Source: CAD feature listing. Evaluate the final solid. Frame: model axes, mm. A direction names the side the tool comes from. Coordinates: 2 decimals unless noted, no trailing zeros. Order: outer loops, then holes, each group sorted by start corner. A loop starts at its lowest first (then second) coordinate and runs counter-clockwise, first axis right, second up.
```python
from build123d import *

# Parameters (mm, degrees)
BOSS_EXTRUDE1_DEPTH      = 2.2
BOSS_EXTRUDE2_DEPTH      = 4.4
BOSS_EXTRUDE2_DEPTH_BACK = 2
SKETCH1_3_R              = 1.1
SKETCH2_R                = 0.7
BOSS_EXTRUDE3_DEPTH      = 0.6
BOSS_EXTRUDE3_TAPER      = 20


with BuildPart() as part:
    # Sketch1 → Boss-Extrude1 (new body)
    with BuildSketch(Plane(origin=(0, 0, 0), x_dir=(1, 0, 0), z_dir=(0, 1, 0))):
        with BuildLine():
            Line((3.782845085, 1.337043166), (3.527238547, 2.290979755))
            ThreePointArc((3.527238547, 2.290979755), (3.480645964, 2.35170039), (3.404764059, 2.361690433))
            Line((3.404764059, 2.361690433), (-0.362346663, 1.352296157))
            ThreePointArc((-0.362346663, 1.352296157), (-1.399770195, -0.025365361), (-0.313114699, -1.364536253))
            Line((-0.313114699, -1.364536253), (-0.385495815, -1.757932966))
            Line((-0.385495815, -1.757932966), (1.229595775, -1.466971493))
            Line((1.229595775, -1.466971493), (0.801769877, -2.8))
            Line((0.801769877, -2.8), (4.601769877, -2.8))
            ThreePointArc((4.601769877, -2.8), (4.884612589, -2.682842712), (5.001769877, -2.4))
            Line((5.001769877, -2.4), (5.001769877, -0.946410162))
            ThreePointArc((5.001769877, -0.946410162), (4.901769877, -0.773205081), (4.701769877, -0.773205081))
            Line((4.701769877, -0.773205081), (4.041625762, -1.154339463))
            ThreePointArc((4.041625762, -1.154339463), (3.81583188, -1.20709678), (3.598705744, -1.125718327))
            add(Edge.make_bspline(
                [(3.668101763, 0.674971994), (3.507811171, 0.443176193), (3.337919583, 0.271573974), (3.416349663, -0.986324141), (3.598705744, -1.125718327)],
                knots=[0.076223888, 0.076223888, 0.076223888, 0.076223888, 0.275181008, 0.474138129, 0.474138129, 0.474138129, 0.474138129], degree=3))
            ThreePointArc((3.668101763, 0.674971994), (3.798353982, 0.993376676), (3.782845085, 1.337043166))
        make_face()
    extrude(amount=BOSS_EXTRUDE1_DEPTH)

    # Sketch1<3> → Boss-Extrude2 (add, two sides: drawn at the far end of the back side and taken through both)
    with BuildSketch(Plane(origin=(0, 0, 0), x_dir=(1, 0, 0), z_dir=(0, 1, 0)).offset(-BOSS_EXTRUDE2_DEPTH_BACK)):
        with Locations(Location((0, 0, 0), (0, 0, 270))):
            Circle(SKETCH1_3_R)
    extrude(amount=BOSS_EXTRUDE2_DEPTH + BOSS_EXTRUDE2_DEPTH_BACK)

    # Sketch2 → Boss-Extrude3 (add)
    with BuildSketch(Plane.XY.offset(2.8)):
        with Locations((2.701769877, 1.2)):
            Circle(SKETCH2_R)
    extrude(amount=BOSS_EXTRUDE3_DEPTH, taper=BOSS_EXTRUDE3_TAPER)


solid = part.part
```
1. Draft query along Z for faces 5 (the flat face through (3.657, 1.085, -1.807)), 6 (the flat face through (1.02, 1.08, 2.12)), 7 (the flat face through (2, 2.2, 1)). Return one class per face: +Z half, -Z half, draft (parallel to the pull), parting line (faces both ways), or undercut.
2. Section query D-D, the plane z = 2.1. Output: boundary loops of the cut face in (x, y), plus the area to 3 significant figures.
3. Section query A-A, the plane x = -0.75. Output: boundary loops of the cut face in (y, z), plus the area to 3 significant figures.
4. Section query C-C, the plane y = 4. Output: boundary loops of the cut face in (x, z).
5. Section query B-B, the plane z = -1. Output: boundary loops of the cut face in (x, y).
6. Access query for faces 1 (the cylindrical face through (1.09, 3.28, -0.14)), 2 (the cylindrical face through (1.09, -1.01, -0.14)), 3 (the flat face through (0.411, 1.085, 1.614)), 4 (the flat face through (5.002, 1, 2)). Directions: +Z, -Z, +X, -X, +Y, -Y. A direction counts if a zero-diameter tool reaches every point of the face in a straight line with its end or side. Return the directions, or none.
7. Contact query for flat-ended pins moving along their axis: P1, Ø2.5, axis at x = 2.5, z = -1, coming from the -Y side; P2, Ø1.5, axis at x = 2.5, z = -0.5, coming from the +Y side; P3, Ø1.5, axis at x = 0, y = 0, coming from the +Z side. Output: stop coordinate, or through.
8. Material intervals for line 1 along Y through (x, z) = (2.5, 1.55); line 2 along Z through (x, y) = (0, -1.5); line 3 along X through (y, z) = (2, 1.1), sorted ascending.
Answer key:
1. face 5: -Z half
1. face 6: undercut
1. face 7: draft
2. outline: (1.03, 0) - (5, 0) - (5, 2.2) - (1.03, 2.2) - close
2. area: 8.75 mm2
3. outline: (-2, -0.8) - (0, -0.8) - (0, -1.18) - (2.2, -1.18) - (2.2, -0.8) - (4.4, -0.8) - (4.4, 0.8) - (2.2, 0.8) - (2.2, 1.18) - (0, 1.18) - (0, 0.8) - (-2, 0.8) - close
3. area: 12.0 mm2
4. outline: circle Ø2.2 at (0, 0)
5. outline: (-0.98, 0) - (-0.46, 0) - (-0.46, -2) - (0.46, -2) - (0.46, 0) - (3.8, 0) - (3.8, 2.2) - (0.46, 2.2) - (0.46, 4.4) - (-0.46, 4.4) - (-0.46, 2.2) - (-0.98, 2.2) - close
6. face 1: +Y
6. face 2: -Y
6. face 3: +Y, -Y
6. face 4: +Z, -Z, +X, +Y, -Y
7. P1: stops at y = 0
7. P2: stops at y = 2.2
7. P3: stops at z = 1.76
8. line 1: y = 0 to 2.2
8. line 2: z = -1.1 to 1.1
8. line 3: x = -0.87 to 3.57, 4.14 to 5
